Can you work these out from the model? Positions are in its coordinate system, mm. Round coordinates to 2 decimals unless told otherwise and drop trailing zeros. Loops run counter-clockwise (first coordinate to the right, second up) from the corner with the lowest first, then second, coordinate; pieces in that order, holes last.
(1) Will these pins go through, and if not, where does the flat tip stop? pin 1 Ø0.6 at (x, z) = (54.5, 1.5) entering from +Y; pin 2 Ø0.6 at (x, z) = (-55.5, 2.5) entering from -Y; pin 3 Ø1 at (y, z) = (-16.5, 2.5) entering from +X.
(2) I want a section at A-A on x = -44.5. Write out the boundary of the cut face in (y, z), plus the area to 3 significant figures.
(3) I want a section at D-D on y = 19. Write out the boundary of the cut face in (x, z).
(4) If I drill on line 1 along Y through (x, z) = (44.5, 1.85); line 2 along Y through (x, z) = (44.5, 0.85); line 3 along X through (y, z) = (-12.5, 1), over which ranges is the centre line in solid material (lowest first)?
(5) I want a section at B-B on z = 2.35. Write out the boundary of the cut face in (x, y).
(6) I want a section at C-C on y = 31.5. Write out the boundary of the cut face in (x, z), plus the area to 3 significant figures.
Autodesk Inventor part; units mm, degrees
ref_plane "YZ Plane" through (0, 0, 0) normal (1, 0, 0) x (0, 1, 0)
ref_plane "XZ Plane" through (0, 0, 0) normal (0, 1, 0) x (-1, 0, 0)
ref_plane "XY Plane" through (0, 0, 0) normal (0, 0, 1) x (1, 0, 0)
sketch "Sketch1" plane through (0, 0, 0) normal (0, 0, 1) x (1, 0, 0)
  line L0 (-49, -36) -> (49, -36)
  line L1 (49, -36) -> (49, 36)
  line L2 (49, 36) -> (-49, 36)
  line L3 (-49, 36) -> (-49, -36)
  line L4 (-49, -36) -> (49, 36) construction
  line L5 (49, -36) -> (-49, 36) construction
  point P0 (0, 0)
  dimension "d0" = 98
  dimension "d1" = 72
extrude "Extrusion1" add sketch "Sketch1" along normal blind 3
sketch "Sketch2" plane through (0, 0, 3) normal (0, 0, 1) x (1, 0, 0)
  circle A0 centre (-44.5, 31.5) radius 2
  line L0 (-68.6, 0) -> (68.6, 0)
  line L1 (0, 50.4) -> (0, -50.4) construction
  circle A1 centre (44.5, 31.5) radius 2
  circle A2 centre (-44.5, -31.5) radius 2
  circle A3 centre (44.5, -31.5) radius 2
  point P0 (0, 0)
  dimension "d4" = 4
  dimension "d5" = 89
  dimension "d6" = 63
extrude "Extrusion2" cut sketch "Sketch2" against normal through all
sketch "Sketch3" plane through (0, 0, 3) normal (0, 0, 1) x (1, 0, 0)
  line L0 (-68.6, 0) -> (68.6, 0) construction
  line L1 (-64, -6) -> (-49, -6)
  line L2 (-49, -6) -> (-49, 6)
  line L3 (-49, 6) -> (-64, 6)
  line L4 (-64, 6) -> (-64, -6)
  line L5 (-64, -6) -> (-49, 6) construction
  line L6 (-49, -6) -> (-64, 6) construction
  line L7 (-49, 36) -> (-49, -36) construction
  line L8 (0, 50.4) -> (0, -50.4)
  line L9 (64, -6) -> (49, -6)
  line L10 (49, -6) -> (49, 6)
  line L11 (49, 6) -> (64, 6)
  line L12 (64, 6) -> (64, -6)
  line L13 (64, -6) -> (49, 6) construction
  line L14 (49, -6) -> (64, 6) construction
  point P0 (0, 0)
  point P1 (-56.5, 0)
  point P2 (-49, 0)
  point P3 (56.5, 0)
  point P4 (49, 0)
  dimension "d9" = 12
  dimension "d10" = 15
extrude "Extrusion3" add sketch "Sketch3" against normal up to surface (3 mm away)
fillet "Fillet1" radius 2 12 edges at (-49, 6, 1.5) (-49, -6, 1.5) (49, -6, 1.5) (49, 6, 1.5) (49, 36, 1.5) (-49, 36, 1.5) (-49, -36, 1.5) (-64, -6, 1.5) (-64, 6, 1.5) (49, -36, 1.5) (64, -6, 1.5) (64, 6, 1.5)
chamfer "Chamfer1" distance 1 angle 45 10 edges at (0, 36, 0) (-48.4142, 35.4142, 0) (-49, 21, 0) (-49, -21, 0) (-48.4142, -35.4142, 0) (0, -36, 0) (48.4142, -35.4142, 0) (49, -21, 0) (49, 21, 0) (48.4142, 35.4142, 0)
sketch "Sketch4" plane through (0, 0, 0) normal (0, 0, -1) x (-1, 0, 0)
  circle A0 centre (-51, -8) radius 1.5
  line L0 (-49, -8) -> (-49, -34)
  line L1 (-62, -6) -> (-51, -6)
  point P0 (0, 0)
  dimension "d17" = 2
  dimension "d18" = 2
  dimension "d19" = 3
equation "\"d18\" = d17"
properties part number "BatteryHolder"
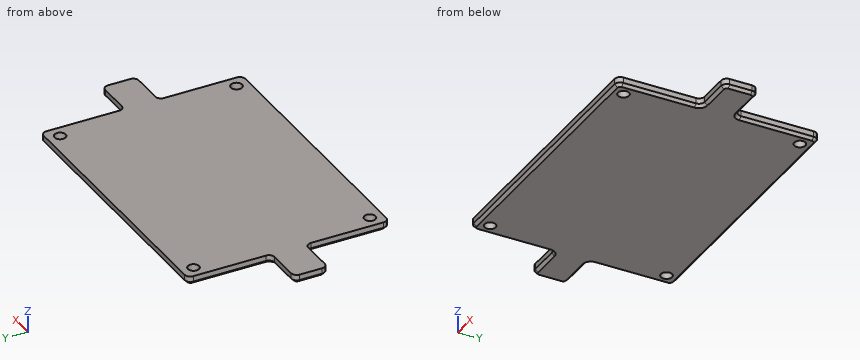
Filled sheet:
1. pin 1: stops at y = 6
1. pin 2: stops at y = -6
1. pin 3: stops at x = 49
2. outline: (-36, 1) - (-35, 0) - (-33.5, 0) - (-33.5, 3) - (-36, 3) - close; (-29.5, 0) - (29.5, 0) - (29.5, 3) - (-29.5, 3) - close; (33.5, 0) - (35, 0) - (36, 1) - (36, 3) - (33.5, 3) - close
2. area: 191 mm2
3. outline: (-49, 1) - (-48, 0) - (48, 0) - (49, 1) - (49, 3) - (-49, 3) - close
4. line 1: y = -36 to -33.5, -29.5 to 29.5, 33.5 to 36
4. line 2: y = -35.85 to -33.5, -29.5 to 29.5, 33.5 to 35.85
4. line 3: x = -49 to 49
5. outline: (-64, -4) arc R2 ccw to (-62, -6) - (-51, -6) arc R2 cw to (-49, -8) - (-49, -34) arc R2 ccw to (-47, -36) - (47, -36) arc R2 ccw to (49, -34) - (49, -8) arc R2 cw to (51, -6) - (62, -6) arc R2 ccw to (64, -4) - (64, 4) arc R2 ccw to (62, 6) - (51, 6) arc R2 cw to (49, 8) - (49, 34) arc R2 ccw to (47, 36) - (-47, 36) arc R2 ccw to (-49, 34) - (-49, 8) arc R2 cw to (-51, 6) - (-62, 6) arc R2 ccw to (-64, 4) - close; hole circle Ø4 at (-44.5, -31.5); hole circle Ø4 at (-44.5, 31.5); hole circle Ø4 at (44.5, -31.5); hole circle Ø4 at (44.5, 31.5)
6. outline: (-49, 1) - (-48, 0) - (-46.5, 0) - (-46.5, 3) - (-49, 3) - close; (-42.5, 0) - (42.5, 0) - (42.5, 3) - (-42.5, 3) - close; (46.5, 0) - (48, 0) - (49, 1) - (49, 3) - (46.5, 3) - close
6. area: 269 mm2
